from build123d import *

# Parameters (mm, degrees)
CUT_EXTRUDE1_DEPTH = 223.822799552
CUT_EXTRUDE2_DEPTH = 223.822799552


with BuildPart() as part:
    # Sketch1 → Revolve1 (revolve)
    with BuildSketch(Plane(origin=(0, 0, 0), x_dir=(0, 0, -1), z_dir=(1, 0, 0))):
        Polygon((13.36858006, 0), (155, 0), (155, 5), (150, 5), (150, 15), (155, 15), (155, 25), (150, 25), (150, 35), (155, 35), (155, 40), (13.36858006, 40), align=None)
    revolve(axis=Axis((0, 0, 0), (0, 1, 0)))

    # Sketch2 → Cut-Extrude1 (cut, through all)
    with BuildSketch(Plane.XZ):
        with BuildLine():
            Line((-4, 16.756133146), (4, 16.756133146))
            Line((4, 16.756133146), (4, 12.756133146))
            ThreePointArc((4, 12.756133146), (0, 13.36858006), (-4, 12.756133146))
            Line((-4, 12.756133146), (-4, 16.756133146))
        make_face()
    extrude(amount=-CUT_EXTRUDE1_DEPTH, mode=Mode.SUBTRACT)

    # Sketch3 → Cut-Extrude2 (cut, through all)
    with BuildSketch(Plane.XZ):
        with BuildLine():
            Line((0, 29.580398915), (0, 134.82214713))
            ThreePointArc((0, 134.82214713), (1.530598787, 138.422599216), (5.18530209, 139.818712264))
            ThreePointArc((5.18530209, 139.818712264), (35.071098816, 135.448062683), (63.322556568, 124.765433861))
            ThreePointArc((63.322556568, 124.765433861), (65.852633094, 121.73068432), (65.389787061, 117.806813075))
            Line((65.389787061, 117.806813075), (12.582866204, 26.34254316))
            ThreePointArc((12.582866204, 26.34254316), (10.127088699, 24.207156024), (6.877282654, 24.035452633))
            ThreePointArc((6.877282654, 24.035452633), (5.530526507, 24.380592211), (4.166666667, 24.65033243))
            ThreePointArc((4.166666667, 24.65033243), (1.181186921, 26.352912794), (0, 29.580398915))
        make_face()
        with BuildLine():
            Line((25.617376915, 14.790199458), (116.759404407, 67.411073565))
            ThreePointArc((116.759404407, 67.411073565), (120.642786773, 67.885762175), (123.67920779, 65.418752795))
            ThreePointArc((123.67920779, 65.418752795), (134.837012585, 37.351568828), (139.711313522, 7.543774309))
            ThreePointArc((139.711313522, 7.543774309), (138.348181588, 3.835288995), (134.718586392, 2.274189795))
            Line((134.718586392, 2.274189795), (29.104744679, 2.274189795))
            ThreePointArc((29.104744679, 2.274189795), (26.027556419, 3.333261933), (24.253953899, 6.061824829))
            ThreePointArc((24.253953899, 6.061824829), (23.879475467, 7.400719654), (23.431147429, 8.716727032))
            ThreePointArc((23.431147429, 8.716727032), (23.412885403, 12.153518517), (25.617376915, 14.790199458))
        make_face()
        with BuildLine():
            Line((25.617376915, -14.790199458), (116.759404407, -67.411073565))
            ThreePointArc((116.759404407, -67.411073565), (119.112187985, -70.536837041), (118.4939057, -74.399959468))
            ThreePointArc((118.4939057, -74.399959468), (99.765913769, -98.096493855), (76.388756953, -117.221659551))
            ThreePointArc((76.388756953, -117.221659551), (72.495548494, -117.895395325), (69.328799331, -115.53262328))
            Line((69.328799331, -115.53262328), (16.521878475, -24.068353365))
            ThreePointArc((16.521878475, -24.068353365), (15.900467721, -20.873894091), (17.376671245, -17.973627804))
            ThreePointArc((17.376671245, -17.973627804), (18.348948961, -16.979872557), (19.264480762, -15.933605397))
            ThreePointArc((19.264480762, -15.933605397), (22.231698483, -14.199394277), (25.617376915, -14.790199458))
        make_face()
        with BuildLine():
            Line((0, -29.580398915), (0, -134.82214713))
            ThreePointArc((0, -134.82214713), (-1.530598787, -138.422599216), (-5.18530209, -139.818712264))
            ThreePointArc((-5.18530209, -139.818712264), (-35.071098816, -135.448062683), (-63.322556568, -124.765433861))
            ThreePointArc((-63.322556568, -124.765433861), (-65.852633094, -121.73068432), (-65.389787061, -117.806813075))
            Line((-65.389787061, -117.806813075), (-12.582866204, -26.34254316))
            ThreePointArc((-12.582866204, -26.34254316), (-10.127088699, -24.207156024), (-6.877282654, -24.035452633))
            ThreePointArc((-6.877282654, -24.035452633), (-5.530526507, -24.380592211), (-4.166666667, -24.65033243))
            ThreePointArc((-4.166666667, -24.65033243), (-1.181186921, -26.352912794), (0, -29.580398915))
        make_face()
        with BuildLine():
            Line((-25.617376915, -14.790199458), (-116.759404407, -67.411073565))
            ThreePointArc((-116.759404407, -67.411073565), (-120.642786773, -67.885762175), (-123.67920779, -65.418752795))
            ThreePointArc((-123.67920779, -65.418752795), (-134.837012585, -37.351568828), (-139.711313522, -7.543774309))
            ThreePointArc((-139.711313522, -7.543774309), (-138.348181588, -3.835288995), (-134.718586392, -2.274189795))
            Line((-134.718586392, -2.274189795), (-29.104744679, -2.274189795))
            ThreePointArc((-29.104744679, -2.274189795), (-26.027556419, -3.333261933), (-24.253953899, -6.061824829))
            ThreePointArc((-24.253953899, -6.061824829), (-23.879475467, -7.400719654), (-23.431147429, -8.716727032))
            ThreePointArc((-23.431147429, -8.716727032), (-23.412885403, -12.153518517), (-25.617376915, -14.790199458))
        make_face()
        with BuildLine():
            Line((-25.617376915, 14.790199458), (-116.759404407, 67.411073565))
            ThreePointArc((-116.759404407, 67.411073565), (-119.112187985, 70.536837041), (-118.4939057, 74.399959468))
            ThreePointArc((-118.4939057, 74.399959468), (-99.765913769, 98.096493855), (-76.388756953, 117.221659551))
            ThreePointArc((-76.388756953, 117.221659551), (-72.495548494, 117.895395325), (-69.328799331, 115.53262328))
            Line((-69.328799331, 115.53262328), (-16.521878475, 24.068353365))
            ThreePointArc((-16.521878475, 24.068353365), (-15.900467721, 20.873894091), (-17.376671245, 17.973627804))
            ThreePointArc((-17.376671245, 17.973627804), (-18.348948961, 16.979872557), (-19.264480762, 15.933605397))
            ThreePointArc((-19.264480762, 15.933605397), (-22.231698483, 14.199394277), (-25.617376915, 14.790199458))
        make_face()
    extrude(amount=-CUT_EXTRUDE2_DEPTH, mode=Mode.SUBTRACT)


solid = part.part
Check sheet for the modelled part. Datum: model origin and axes. Units: mm. Round coordinates to 2 decimals unless told otherwise and drop trailing zeros. Order: outer loops, then holes, each group sorted by start corner. A loop starts at its lowest first (then second) coordinate and runs counter-clockwise, first axis right, second up.
(1) Cross-section at D-D, the plane z = 89. Enter the section's corners in (x, y), and give its area (3 significant figures).
(2) Scan lines: probe 1 along X at (y, z) = (37.5, -46.5); probe 2 along Z at (x, y) = (-52, 16); probe 3 along Z at (x, y) = (-74.5, 18.5). Record each from-to range of solid material in increasing order.
(3) Cross-section at A-A, the plane x = -130.5. Enter the section's corners in (y, z).
(4) Go/stop test with flat-tipped pins: P1, Ø3, axis at y = 21.5, z = 122.5, coming from the +X side; P2, Ø1.5, axis at y = 5.5, z = 57.5, coming from the +X side; P3, Ø20, axis at y = 28.5, z = 108.5, coming from the +X side; P4, Ø21.5, axis at x = 0, z = 0, coming from the -Y side. Record where each tip stops, or that it passes through.
(5) Cross-section at B-B, the plane z = -53.5. State how many separate pieces and enclosed holes the cut face has, and give its area (3 significant figures).
(6) Draft check along X on faces 1 (the flat face through (-39.356, 19.72, -72.715)), 2 (the cylindrical face through (-34.661, 19.72, -135.554)), 3 (the flat face through (-127, 15, -81)), 4 (the cylindrical face through (151.314, 2.535, 33.601)). Enter one of: pulls with the +X half, pulls with the -X half, needs draft (parallel to the pull), parting line crosses it, or undercut.
Check sheet entries:
1. outline: (-126.9, 0) - (-107.96, 0) - (-107.96, 40) - (-126.9, 40) - (-126.9, 35) - (-120.74, 35) - (-120.74, 25) - (-126.9, 25) - (-126.9, 15) - (-120.74, 15) - (-120.74, 5) - (-126.9, 5) - close; (-54.01, 0) - (0, 0) - (0, 40) - (-54.01, 40) - close; (48.76, 0) - (126.9, 0) - (126.9, 5) - (120.74, 5) - (120.74, 15) - (126.9, 15) - (126.9, 25) - (120.74, 25) - (120.74, 35) - (126.9, 35) - (126.9, 40) - (48.76, 40) - close
1. area: 5,800 mm2
2. probe 1: x = -147.86 to -131.96, -80.54 to -24.22, 0 to 29.47, 80.54 to 147.86
2. probe 2: z = -146.02 to -129.89, -94.62 to -30.02, -2.27 to 30.02, 85.52 to 146.02
2. probe 3: z = -135.92 to -43.01, -2.27 to 43.01, 117.96 to 135.92
3. outline: (0, -83.63) - (5, -83.63) - (5, -73.96) - (15, -73.96) - (15, -83.63) - (25, -83.63) - (25, -73.96) - (35, -73.96) - (35, -83.63) - (40, -83.63) - (40, -50.46) - (0, -50.46) - close; (0, -2.27) - (40, -2.27) - (40, 83.63) - (35, 83.63) - (35, 73.96) - (25, 73.96) - (25, 83.63) - (15, 83.63) - (15, 73.96) - (5, 73.96) - (5, 83.63) - (0, 83.63) - close
4. P1: stops at x = 96.87
4. P2: stops at x = 144.16
4. P3: stops at x = 119.15
4. P4: passes through
5. separate pieces: 4
5. enclosed holes: 0
5. area: 6,460 mm2
6. face 1: undercut
6. face 2: undercut
6. face 3: needs draft
6. face 4: parting line crosses it
